from build123d import *

# Parameters (mm, degrees)
BOX077_W               = 11.5
BOX077_H               = 10.95
BOX077_DEPTH           = 1.05
BOX076_W               = 11.5
BOX076_H               = 11
BOX076_DEPTH           = 1.15
CUT024_PLACEMENT_ANGLE = 270


with BuildPart() as small_cu_gnd_electrode022:
    # Box077 → Box077 (new body)
    with BuildSketch(Plane.XY.offset(0.05)):
        with Locations((5.75, 5.475)):
            Rectangle(BOX077_W, BOX077_H)
    extrude(amount=BOX077_DEPTH)


with BuildPart() as large_cu_electrode_short_axis_gnd002:
    # Box076 → Box076 (new body)
    with BuildSketch(Plane.XY):
        with Locations((5.75, 5.5)):
            Rectangle(BOX076_W, BOX076_H)
    extrude(amount=BOX076_DEPTH)

    # Cut024: cut Small Cu GND Electrode022
    add(small_cu_gnd_electrode022.part, mode=Mode.SUBTRACT)


with BuildPart() as large_cu_electrode_short_axis_gnd002_1:
    # Cut024 placement: moved
    add(large_cu_electrode_short_axis_gnd002.part.moved(Location((-4.76, 21.13, 20.55))).rotate(Axis((-4.76, 21.13, 20.55), (0, 0, 1)), CUT024_PLACEMENT_ANGLE))


solid = large_cu_electrode_short_axis_gnd002_1.part
Here's how the part is built. I have some questions about the finished solid (model axes, mm). Give positions to 0.01 mm unless a question says otherwise; leave off trailing zeros. Write each loop counter-clockwise with the first axis right and the second up, starting at its lowest first coordinate (ties: lowest second). Pieces come first, ordered by that corner, then holes. Notation, with made-up numbers: (-7, -31.5) -> (18, -31.5) arc R12 cw to (18, -14.5) -> close; hole circle Ø2 at (-14.5, 15). An arc over 180 degrees is marked (long way). Use one line per item in the form item = value. Start each with the question number.
1. Imagine slicing it at B-B on x = 4.5. List the corners of the cut face in (y, z) for me, plus the area to 3 significant figures.
2. Imagine slicing it at A-A on y = 19.75. List the corners of the cut face in (x, z) for me, plus the area to 3 significant figures.
3. Will this pin go through, and if not, where does the flat tip stop? pin 1 Ø0.5 at (y, z) = (13.5, 21) entering from -X.
4. Imagine slicing it at C-C on z = 20.9. List the corners of the cut face in (x, y) for me, plus the area to 3 significant figures.
Entries:
q1.outline = (9.63, 20.55) -> (21.13, 20.55) -> (21.13, 20.6) -> (9.63, 20.6) -> close; (9.63, 21.65) -> (21.13, 21.65) -> (21.13, 21.7) -> (9.63, 21.7) -> close
q1.area = 1.15 mm²
q2.outline = (-4.76, 20.55) -> (6.24, 20.55) -> (6.24, 21.7) -> (-4.76, 21.7) -> (-4.76, 21.65) -> (6.19, 21.65) -> (6.19, 20.6) -> (-4.76, 20.6) -> close
q2.area = 1.15 mm²
q3.pin_1 = 6.19
q4.outline = (6.19, 9.63) -> (6.24, 9.63) -> (6.24, 21.13) -> (6.19, 21.13) -> close
q4.area = 0.575 mm²
